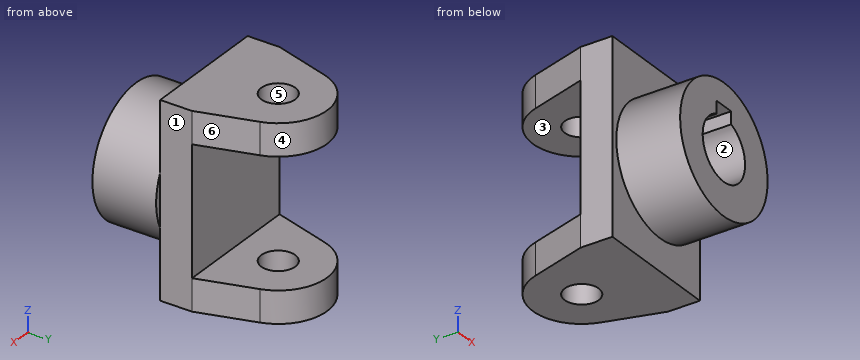
from build123d import *

# Parameters (mm, degrees)
SKETCH1_R           = 8
BOSS_EXTRUDE2_DEPTH = 15
SKETCH1_5_W         = 60
SKETCH1_5_H         = 15
BOSS_EXTRUDE3_DEPTH = 90
BOSS_EXTRUDE4_START = -15
SKETCH2_R           = 8
BOSS_EXTRUDE4_DEPTH = 15
SKETCH3_R           = 30
BOSS_EXTRUDE5_DEPTH = 30


with BuildPart() as part:
    # Sketch1 → Boss-Extrude2 (new body)
    with BuildSketch(Plane.XY):
        with BuildLine():
            Line((30, -20), (22.03289839, 6.599347585))
            ThreePointArc((22.03289839, 6.599347585), (0, 23), (-22.03289839, 6.599347585))
            Line((-22.03289839, 6.599347585), (-30, -20))
            Line((-30, -20), (30, -20))
        make_face()
        Circle(SKETCH1_R, mode=Mode.SUBTRACT)
    extrude(amount=BOSS_EXTRUDE2_DEPTH)

    # Sketch1_5 → Boss-Extrude3 (add)
    with BuildSketch(Plane.XY):
        with Locations((0, -27.5)):
            Rectangle(SKETCH1_5_W, SKETCH1_5_H)
    extrude(amount=BOSS_EXTRUDE3_DEPTH)

    # Sketch2 → Boss-Extrude4 (add)
    with BuildSketch(Plane.XY.offset(90).offset(BOSS_EXTRUDE4_START)):
        with BuildLine():
            Line((30, -20), (22.03289839, 6.599347585))
            ThreePointArc((22.03289839, 6.599347585), (0, 23), (-22.03289839, 6.599347585))
            Line((-22.03289839, 6.599347585), (-30, -20))
            Line((-30, -20), (30, -20))
        make_face()
        Circle(SKETCH2_R, mode=Mode.SUBTRACT)
    extrude(amount=BOSS_EXTRUDE4_DEPTH)

    # Sketch3 → Boss-Extrude5 (add)
    with BuildSketch(Plane.XZ.offset(35)):
        with Locations(Location((2.720866767, 44.917667838, 0), (0, 0, 24.59059327))):
            Circle(SKETCH3_R)
        with BuildLine():
            Line((-2.279133233, 58.561813924), (-2.279133233, 64.417667838))
            Line((-2.279133233, 64.417667838), (7.720866767, 64.417667838))
            Line((7.720866767, 64.417667838), (7.720866767, 58.561813924))
            ThreePointArc((7.720866767, 58.561813924), (2.720866767, 30.386228736), (-2.279133233, 58.561813924))
        make_face(mode=Mode.SUBTRACT)
    extrude(amount=BOSS_EXTRUDE5_DEPTH)


solid = part.part
The listing builds one solid part. Answer for the finished solid, in the listing's coordinates (mm). Face numbers are marked on the shaded views. A direction names the side the tool comes from. Round coordinates to 2 decimals unless told otherwise and drop trailing zeros. Write each loop counter-clockwise with the first axis right and the second up, starting at its lowest first coordinate (ties: lowest second). Pieces come first, ordered by that corner, then holes. Notation, with made-up numbers: M 34.5,5.25 L 80.5,5.25 A17 cw 80.5,21.25 Z; hole C 67.5,18.25 d2. An arc over 180 degrees is marked long. Write each question's results on one line, items separated by ' | '. Start each with the question number.
Item 1: Which of the six approach directions +Z, -Z, +X, -X, +Y, -Y give full straight-line access (tool end or side, diameter ignored) to the marked faces 1, 2 and 3?
Item 2: Find section D-D on x = 0. Write down the section's boundary in (y, z).
Item 3: The mould has two halves that part along X. Classify the marked faces 4, 5 and 6: +X half, -X half, draft (parallel to the pull), parting line (faces both ways), or undercut.
Item 4: Straight lines are drawn through the part: probe 1 along Z at (x, y) = (-8, -6); probe 2 along Y at (x, z) = (10, 24); probe 3 along Y at (x, z) = (-21, 63.5). For each, find the intervals that lie inside material, in ascending order.
Item 5: Find section A-A on z = 76.5. Write down the section's boundary in (x, y), and give its area (3 significant figures).
Item 6: Given pin 1 Ø1.8 at (y, z) = (-44.5, 61.5) entering from +X; pin 2 Ø1 at (x, z) = (-9.5, 20) entering from +Y; pin 3 Ø4.5 at (y, z) = (-45, 63) entering from -X, each flat-ended and moving along its own axis, determine where each tip first touches the part or whether it passes through.
Item 7: Find section C-C on y = 0. Write down the section's boundary in (x, z).
Item 8: Find section B-B on y = -10. Write down the section's boundary in (x, z), and give its area (3 significant figures).
Answer block:
1) face 1: +Z, -Z, +X, +Y | face 2: -Y | face 3: +X, -X, +Y
2) outline: M -65,15.04 L -35,15.04 L -35,0 L -8,0 L -8,15 L -20,15 L -20,75 L -8,75 L -8,90 L -35,90 L -35,74.79 L -65,74.79 L -65,64.42 L -35,64.42 L -35,30.64 L -65,30.64 Z; M 8,0 L 23,0 L 23,15 L 8,15 Z; M 8,75 L 23,75 L 23,90 L 8,90 Z
3) face 4: parting line | face 5: undercut | face 6: +X half
4) probe 1: z = 0 to 15, 75 to 90 | probe 2: y = -65 to -20 | probe 3: y = -35 to -20
5) outline: M -30,-35 L 30,-35 L 30,-20 L 22.03,6.6 A23 ccw -22.03,6.6 L -30,-20 Z; hole C 0,0 d16 | area: 2,610 mm²
6) pin 1: stops at x = 28.3 | pin 2: stops at y = -20 | pin 3: stops at x = -22.76
7) outline: M -24.01,0 L -8,0 L -8,15 L -24.01,15 Z; M -24.01,75 L -8,75 L -8,90 L -24.01,90 Z; M 8,0 L 24.01,0 L 24.01,15 L 8,15 Z; M 8,75 L 24.01,75 L 24.01,90 L 8,90 Z
8) outline: M -27,0 L 27,0 L 27,15 L -27,15 Z; M -27,75 L 27,75 L 27,90 L -27,90 Z | area: 1,620 mm²
